```python
from build123d import *

# Parameters (mm, degrees)
CROQUIS1_W              = 20
CROQUIS1_H              = 20
SALIENTE_EXTRUIR1_DEPTH = 13
CROQUIS3_W              = 13.3
CROQUIS3_H              = 2.6
CORTAR_EXTRUIR1_DEPTH   = 18
CORTAR_EXTRUIR2_REACH   = 33.129
CROQUIS4_R              = 5


with BuildPart() as part:
    # Croquis1 → Saliente-Extruir1 (new body)
    with BuildSketch(Plane(origin=(0, 0, 0), x_dir=(1, 0, 0), z_dir=(0, 1, 0))):
        with Locations((-10, -10)):
            Rectangle(CROQUIS1_W, CROQUIS1_H)
    extrude(amount=SALIENTE_EXTRUIR1_DEPTH)

    # Croquis3 → Cortar-Extruir1 (cut)
    with BuildSketch(Plane.XY.offset(20)):
        with Locations((-10, 8.7)):
            Rectangle(CROQUIS3_W, CROQUIS3_H)
    extrude(amount=-CORTAR_EXTRUIR1_DEPTH, mode=Mode.SUBTRACT)

    # Cortar-Extruir2: up to this face of the body (flat: up to its plane)
    cortar_extruir2_end = Plane(part.part.faces().sort_by_distance((-10, 0, 10))[0])
    # Croquis4 → Cortar-Extruir2 (cut, up to the picked face)
    with BuildSketch(Plane(origin=(0, 13, 0), x_dir=(1, 0, 0), z_dir=(0, 1, 0)), mode=Mode.PRIVATE) as cortar_extruir2_sk1:
        with Locations(Location((-10, -11, 0), (0, 0, 90))):
            Circle(CROQUIS4_R)
    cortar_extruir2_tool1 = split(extrude(cortar_extruir2_sk1.sketch, amount=-CORTAR_EXTRUIR2_REACH, mode=Mode.PRIVATE), bisect_by=cortar_extruir2_end, keep=Keep.BOTH, mode=Mode.PRIVATE)
    add(cortar_extruir2_tool1.solids().sort_by(Axis((-10, 13, 11), (0, -1, 0)))[0], mode=Mode.SUBTRACT)


solid = part.part
```
Geometry check sheet. Reference: the model listing, model coordinates, mm. A direction names the side the tool comes from. Coordinates: 2 decimals unless noted, no trailing zeros. Write each loop counter-clockwise with the first axis right and the second up, starting at its lowest first coordinate (ties: lowest second). Pieces come first, ordered by that corner, then holes. Notation, with made-up numbers: M 17.25,-6 L 54.25,-6 A28 ccw 54.25,21 Z; hole C 75.5,42.25 d7. An arc over 180 degrees is marked long. One line per item, written item: value. Start each with the question number.
(1) Tool access check on faces 1 (the face through (-10, 0, 5)), 2 (the face through (-15, 7.4, 13)). Record the directions out of +Z, -Z, +X, -X, +Y, -Y that give a thin tool (end or side, any length) a straight path to the whole face; none if there is none.
(2) Sectioned sample at C-C, the plane z = 16.5. Enter the section's corners in (x, y).
(3) Release check for a two-part mould opening along Z. For faces 3 (the face through (-3.35, 9, 11)), 4 (the face through (-11.5, 11.52, 6.23)), 5 (the face through (-10, 6, 0)) record: released by +Z, released by -Z, zero draft, split by the parting line, or undercut.
(4) Sectioned sample at A-A, the plane z = 11. Enter the section's corners in (x, y), and give its area (3 significant figures).
(5) Scan lines: line 1 along Y through (x, z) = (-16, 5.5); line 2 along X through (y, z) = (4.5, 11); line 3 along X through (y, z) = (9, 8.5). Record each from-to range of solid material in increasing order. Write a range as [from, to].
(6) Depth check by flat-ended pin: pin 1 (1 mm diameter, centred on x = -9.5, z = 15, fed in from +Y). Enter the tip coordinate at first touch or a pass-through.
(7) Sectioned sample at B-B, the plane x = -10. Enter the section's corners in (y, z), and give its area (3 significant figures).
(8) Sectioned sample at D-D, the plane y = 10.5. Enter the section's corners in (x, z), and give its area (3 significant figures).
Filled sheet:
1. face 1: +Z, -Z, +X, -X, -Y
1. face 2: +Z
2. outline: M -20,0 L 0,0 L 0,13 L -20,13 Z; hole M -16.65,7.4 L -3.35,7.4 L -3.35,10 L -16.65,10 Z
3. face 3: zero draft
3. face 4: undercut
3. face 5: released by -Z
4. outline: M -20,0 L -15,0 L -15,7.4 L -16.65,7.4 L -16.65,10 L -15,10 L -15,13 L -20,13 Z; M -5,0 L 0,0 L 0,13 L -5,13 L -5,10 L -3.35,10 L -3.35,7.4 L -5,7.4 Z
4. area: 121 mm²
5. line 1: [0, 7.4], [10, 13]
5. line 2: [-20, -15], [-5, 0]
5. line 3: [-20, -16.65], [-3.35, 0]
6. pin 1: through
7. outline: M 0,0 L 13,0 L 13,6 L 10,6 L 10,2 L 7.4,2 L 7.4,6 L 0,6 Z; M 0,16 L 7.4,16 L 7.4,20 L 0,20 Z; M 10,16 L 13,16 L 13,20 L 10,20 Z
7. area: 109 mm²
8. outline: M -20,0 L 0,0 L 0,20 L -20,20 Z; hole C -10,11 d10
8. area: 321 mm²
